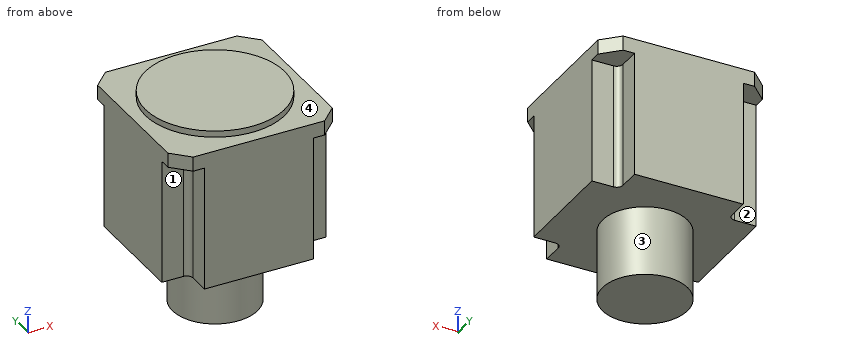
```python
from build123d import *

# Parameters (mm, degrees)
EXTRUDE_1_DEPTH = 11.5
SKETCH_2_R      = 55
EXTRUDE_2_DEPTH = 5
SKETCH_5_W      = 86
SKETCH_5_H      = 22
SKETCH_5_W_2    = 22
SKETCH_5_H_2    = 86
EXTRUDE_4_DEPTH = 98.5
FILLET_1_R      = 5
SKETCH_6_R      = 33.6
EXTRUDE_5_DEPTH = 55


with BuildPart() as part:
    # 草图1 → 凸台-拉伸1 (new body)
    with BuildSketch(Plane.XY):
        Polygon((-65, -52), (-52, -65), (52, -65), (65, -52), (65, 52), (52, 65), (-52, 65), (-65, 52), align=None)
    extrude(amount=EXTRUDE_1_DEPTH)

    # 草图2 → 凸台-拉伸2 (add)
    with BuildSketch(Plane.XY.offset(11.5)):
        Circle(SKETCH_2_R)
    extrude(amount=EXTRUDE_2_DEPTH)

    # 草图5 → 凸台-拉伸4 (add)
    with BuildSketch(Plane(origin=(0, 0, 0), x_dir=(-1, 0, 0), z_dir=(0, 0, -1))):
        with Locations((0, 54)):
            Rectangle(SKETCH_5_W, SKETCH_5_H)
        with Locations((-54, 0)):
            Rectangle(SKETCH_5_W_2, SKETCH_5_H_2)
        Rectangle(SKETCH_5_W, SKETCH_5_H_2)
        with Locations((54, 0)):
            Rectangle(SKETCH_5_W_2, SKETCH_5_H_2)
        with Locations((0, -54)):
            Rectangle(SKETCH_5_W, SKETCH_5_H)
    extrude(amount=EXTRUDE_4_DEPTH)

    # 圆角1
    fillet_1_edges = [part.edges().sort_by_distance(p)[0] for p in [
        (43, 43, -49.25),
        (43, -43, -49.25),
        (-43, -43, -49.25),
        (-43, 43, -49.25),
    ]]
    fillet(fillet_1_edges, radius=FILLET_1_R)

    # 草图6 → 凸台-拉伸5 (add)
    with BuildSketch(Plane(origin=(0, 0, -98.5), x_dir=(-1, 0, 0), z_dir=(0, 0, -1))):
        Circle(SKETCH_6_R)
    extrude(amount=EXTRUDE_5_DEPTH)


solid = part.part
```
Design review of the part built by this model. Coordinates are the model's own, in mm. Face numbers are marked on the shaded views. A direction names the side the tool comes from. Coordinates: 2 decimals unless noted, no trailing zeros. Write each loop counter-clockwise with the first axis right and the second up, starting at its lowest first coordinate (ties: lowest second). Pieces come first, ordered by that corner, then holes.
1) Insertion check: pin 1 (11 mm diameter, centred on x = 52, y = -52.5, fed in from -Z); pin 2 (8.5 mm diameter, centred on y = 60.5, z = -60, fed in from +X); pin 3 (8.5 mm diameter, centred on y = -54.5, z = -66.5, fed in from -X). Each pin has a flat end and moves straight along its axis. Give the tip position at first contact, or say it passes through.
2) To check wall thickness, follow L1, parallel to Z at x = 7, y = 59.5; L2, parallel to Z at x = -16, y = -52; L3, parallel to X at y = -51, z = -35. State the ranges of each line that lie inside material, in increasing order.
3) Add section A-A (x = 57.5). Write out the cut boundary in (y, z), plus the area to 3 significant figures.
4) Add section C-C (z = 6). Write out the cut boundary in (x, y).
5) Add section B-B (y = 0). Write out the cut boundary in (x, z).
6) Machinability: for the marked faces 1, 2, 3 and 4, which of the approach directions +Z, -Z, +X, -X, +Y, -Y give a long, thin tool a straight path to every point of the face, cutting with its end or side? Answer none if there is none.
Check result:
1. pin 1: stops at z = 0
1. pin 2: stops at x = 43
1. pin 3: stops at x = -43
2. L1: z = -98.5 to 11.5
2. L2: z = -98.5 to 16.5
2. L3: x = -43 to 43
3. outline: (-59.5, 0) - (-43, 0) - (-43, -98.5) - (43, -98.5) - (43, 0) - (59.5, 0) - (59.5, 11.5) - (-59.5, 11.5) - close
3. area: 9,840 mm2
4. outline: (-65, -52) - (-52, -65) - (52, -65) - (65, -52) - (65, 52) - (52, 65) - (-52, 65) - (-65, 52) - close
5. outline: (-65, -98.5) - (-33.6, -98.5) - (-33.6, -153.5) - (33.6, -153.5) - (33.6, -98.5) - (65, -98.5) - (65, 11.5) - (55, 11.5) - (55, 16.5) - (-55, 16.5) - (-55, 11.5) - (-65, 11.5) - close
6. face 1: -Z, -X, -Y
6. face 2: -Z, -X, +Y
6. face 3: -Z
6. face 4: +Z
